Part model, mm, in its own coordinate system. Give positions to 0.01 mm unless a question says otherwise; leave off trailing zeros. One line per item, written item: value.
```python
from build123d import *

# Parameters (mm, degrees)
SKETCH1_W                                         = 357.94
SKETCH1_H                                         = 550
BOSS_EXTRUDE1_DEPTH                               = 16
CSK_FOR_4_FLAT_HEAD_MACHINE_SCREW_100_D           = 3.2639
CSK_FOR_4_FLAT_HEAD_MACHINE_SCREW_100_DEPTH       = 16
CSK_FOR_4_FLAT_HEAD_MACHINE_SCREW_100_CSINK_D     = 5.715
CSK_FOR_4_FLAT_HEAD_MACHINE_SCREW_100_CSINK_ANGLE = 100
LPATTERN1_COUNT                                   = 4
LPATTERN1_PITCH                                   = 176.5
MIRROR1_COPY_1_D                                  = 3.2639
MIRROR1_COPY_1_DEPTH                              = 16
MIRROR1_COPY_1_CSINK_D                            = 5.715
MIRROR1_COPY_1_CSINK_ANGLE                        = 100
MIRROR1_COPY_2_D                                  = 3.2639
MIRROR1_COPY_2_DEPTH                              = 16
MIRROR1_COPY_2_CSINK_D                            = 5.715
MIRROR1_COPY_2_CSINK_ANGLE                        = 100
MIRROR1_COPY_3_D                                  = 3.2639
MIRROR1_COPY_3_DEPTH                              = 16
MIRROR1_COPY_3_CSINK_D                            = 5.715
MIRROR1_COPY_3_CSINK_ANGLE                        = 100


with BuildPart() as part:
    # Sketch1 → Boss-Extrude1 (new body)
    with BuildSketch(Plane.XY):
        Rectangle(SKETCH1_W, SKETCH1_H)
    extrude(amount=BOSS_EXTRUDE1_DEPTH)

    # CSK for #4 Flat Head Machine Screw (100)1
    with Locations(Plane(origin=(-170.97, -265, 16), x_dir=(1, 0, 0), z_dir=(0, 0, 1))):
        with Locations((0, 0)):
            csk_for_4_flat_head_machine_screw_100 = CounterSinkHole(CSK_FOR_4_FLAT_HEAD_MACHINE_SCREW_100_D / 2, CSK_FOR_4_FLAT_HEAD_MACHINE_SCREW_100_CSINK_D / 2, depth=CSK_FOR_4_FLAT_HEAD_MACHINE_SCREW_100_DEPTH, counter_sink_angle=CSK_FOR_4_FLAT_HEAD_MACHINE_SCREW_100_CSINK_ANGLE)

    # LPattern1: CSK for #4 Flat Head Machine Screw (100)1 ×4
    with Locations(*[(0, i * LPATTERN1_PITCH, 0) for i in range(1, LPATTERN1_COUNT)]):
        add(csk_for_4_flat_head_machine_screw_100, mode=Mode.SUBTRACT)

    # Mirror1: CSK for #4 Flat Head Machine Screw (100)1 across plane
    add(csk_for_4_flat_head_machine_screw_100.mirror(Plane(origin=(0, 0, 0), x_dir=(0, 0, 1), z_dir=(1, 0, 0))), mode=Mode.SUBTRACT)

    # Mirror1 copy 1
    with Locations(Plane(origin=(170.97, -88.5, 16), x_dir=(-1, 0, 0), z_dir=(0, 0, 1))):
        with Locations((0, 0)):
            CounterSinkHole(MIRROR1_COPY_1_D / 2, MIRROR1_COPY_1_CSINK_D / 2, depth=MIRROR1_COPY_1_DEPTH, counter_sink_angle=MIRROR1_COPY_1_CSINK_ANGLE)

    # Mirror1 copy 2
    with Locations(Plane(origin=(170.97, 88, 16), x_dir=(-1, 0, 0), z_dir=(0, 0, 1))):
        with Locations((0, 0)):
            CounterSinkHole(MIRROR1_COPY_2_D / 2, MIRROR1_COPY_2_CSINK_D / 2, depth=MIRROR1_COPY_2_DEPTH, counter_sink_angle=MIRROR1_COPY_2_CSINK_ANGLE)

    # Mirror1 copy 3
    with Locations(Plane(origin=(170.97, 264.5, 16), x_dir=(-1, 0, 0), z_dir=(0, 0, 1))):
        with Locations((0, 0)):
            CounterSinkHole(MIRROR1_COPY_3_D / 2, MIRROR1_COPY_3_CSINK_D / 2, depth=MIRROR1_COPY_3_DEPTH, counter_sink_angle=MIRROR1_COPY_3_CSINK_ANGLE)


solid = part.part
```
1) Wall check: line 1 along X through (y, z) = (-265, 5.75); line 2 along Y through (x, z) = (-170.97, 10.5). Give the ranges that are in metal, low to high. Write a range as [from, to].
Answer:
line 1: x = [-178.97, -172.6], [-169.34, 169.34], [172.6, 178.97]
line 2: y = [-275, -266.63], [-263.37, -90.13], [-86.87, 86.37], [89.63, 262.87], [266.13, 275]
2) Drop a flat-ended pin along its axis: P1, Ø4, axis at x = -170.97, y = -265, coming from the +Z side. Give the stop position or say it passes through.
Answer:
P1: stops at z = 15.28
3) Two-plate mould, pull along Z, no slides. Class faces 1 (the face through (-3, 4, 16)), 2 (the face through (-3, 4, 0)), 3 (the face through (-3, -275, 8)): pulls with the +Z half, pulls with the -Z half, needs draft (parallel to the pull), parting line crosses it, or undercut.
Answer:
face 1: pulls with the +Z half
face 2: pulls with the -Z half
face 3: needs draft
